from build123d import *

# Parameters (mm, degrees)
SKETCH_1_W          = 143
SKETCH_1_H          = 50
EXTRUDE_1_DEPTH     = 2
FILLET_1_R          = 3
CUT_EXTRUDE_1_DEPTH = 10
SKETCH_7_R          = 1.5
CUT_EXTRUDE_2_DEPTH = 10


with BuildPart() as part:
    # 草图1 → 凸台-拉伸1 (new body)
    with BuildSketch(Plane.XY):
        Rectangle(SKETCH_1_W, SKETCH_1_H)
    extrude(amount=EXTRUDE_1_DEPTH)

    # 圆角1
    fillet_1_edges = [part.edges().sort_by_distance(p)[0] for p in [
        (-71.5, 25, 1),
        (71.5, 25, 1),
        (71.5, -25, 1),
        (-71.5, -25, 1),
    ]]
    fillet(fillet_1_edges, radius=FILLET_1_R)

    # 草图2 → 切除-拉伸1 (cut)
    with BuildSketch(Plane.XY.offset(2)):
        with BuildLine():
            Line((5, 13), (5, -13))
            ThreePointArc((5, -13), (0, -18), (-5, -13))
            Line((-5, -13), (-5, 13))
            ThreePointArc((-5, 13), (0, 18), (5, 13))
        make_face()
        with BuildLine():
            Line((23, 13), (23, -13))
            ThreePointArc((23, -13), (18, -18), (13, -13))
            Line((13, -13), (13, 13))
            ThreePointArc((13, 13), (18, 18), (23, 13))
        make_face()
        with BuildLine():
            Line((41, 13), (41, -13))
            ThreePointArc((41, -13), (36, -18), (31, -13))
            Line((31, -13), (31, 13))
            ThreePointArc((31, 13), (36, 18), (41, 13))
        make_face()
        with BuildLine():
            Line((59, 13), (59, -13))
            ThreePointArc((59, -13), (54, -18), (49, -13))
            Line((49, -13), (49, 13))
            ThreePointArc((49, 13), (54, 18), (59, 13))
        make_face()
        with BuildLine():
            Line((-59, 13), (-59, -13))
            ThreePointArc((-59, -13), (-54, -18), (-49, -13))
            Line((-49, -13), (-49, 13))
            ThreePointArc((-49, 13), (-54, 18), (-59, 13))
        make_face()
        with BuildLine():
            Line((-41, 13), (-41, -13))
            ThreePointArc((-41, -13), (-36, -18), (-31, -13))
            Line((-31, -13), (-31, 13))
            ThreePointArc((-31, 13), (-36, 18), (-41, 13))
        make_face()
        with BuildLine():
            Line((-23, 13), (-23, -13))
            ThreePointArc((-23, -13), (-18, -18), (-13, -13))
            Line((-13, -13), (-13, 13))
            ThreePointArc((-13, 13), (-18, 18), (-23, 13))
        make_face()
    extrude(amount=-CUT_EXTRUDE_1_DEPTH, mode=Mode.SUBTRACT)

    # 草图7 → 切除-拉伸2 (cut)
    with BuildSketch(Plane(origin=(0, 0, 0), x_dir=(-1, 0, 0), z_dir=(0, 0, -1))):
        with Locations((-68.5, -3)):
            Circle(SKETCH_7_R)
        with Locations((-68.5, 17)):
            Circle(SKETCH_7_R)
    cut_extrude_2 = extrude(amount=-CUT_EXTRUDE_2_DEPTH, mode=Mode.SUBTRACT)

    # 镜向2: 切除-拉伸2 across plane
    add(cut_extrude_2.mirror(Plane.ZY), mode=Mode.SUBTRACT)


solid = part.part
Verification items for the finished model (mm, model axes). A direction names the side the tool comes from. Round coordinates to 2 decimals unless told otherwise and drop trailing zeros. Loops run counter-clockwise (first coordinate to the right, second up) from the corner with the lowest first, then second, coordinate; pieces in that order, holes last. Notation, with made-up numbers: (37, -7.75) - (65, -7.75) arc R13 ccw to (65, 1.25) - close; hole circle Ø4 at (13, 86.5). An arc over 180 degrees is marked (long way). Use a Markdown table: item, result. Add a question column.
1. Access from +Z, -Z, +X, -X, +Y, -Y to the whole of each face (thin tool, end or side, straight path). Record for faces 1 (the face through (-1, 23, 0)), 2 (the face through (36, 18, 1)).
2. Section check D-D, the plane x = 35. Record the boundary of the cut face in (y, z), plus the area to 3 significant figures.
3. Thickness scan on probe 1 along Y at (x, z) = (68.5, 1.2); probe 2 along Y at (x, z) = (36.5, 1.6); probe 3 along Y at (x, z) = (32, 1.5). Record the ranges inside material, lowest first. Write a range as [from, to].
4. Section check B-B, the plane z = 1.3. Give the number of separate pieces and of enclosed holes in the cut face, plus the area to 3 significant figures.
5. Release check for a two-part mould opening along Y. For faces 3 (the face through (70.6, -24.14, 1.01)), 4 (the face through (70.64, 24.1, 1.01)), 5 (the face through (54, 18, 1)) record: released by +Y, released by -Y, zero draft, split by the parting line, or undercut.
6. Section check A-A, the plane x = -18. Record the boundary of the cut face in (y, z).
Checks:
| question | item | result |
|---|---|---|
| 1 | face 1 | -Z, +X, -X, +Y, -Y |
| 1 | face 2 | +Z, -Z |
| 2 | outline | (-25, 0) - (-17.9, 0) - (-17.9, 2) - (-25, 2) - close; (17.9, 0) - (25, 0) - (25, 2) - (17.9, 2) - close |
| 2 | area | 28.4 mm^2 |
| 3 | probe 1 | y = [-25, -4.5], [-1.5, 15.5], [18.5, 25] |
| 3 | probe 2 | y = [-25, -17.97], [17.97, 25] |
| 3 | probe 3 | y = [-25, -16], [16, 25] |
| 4 | separate pieces | 1 |
| 4 | enclosed holes | 11 |
| 4 | area | 4,740 mm^2 |
| 5 | face 3 | released by -Y |
| 5 | face 4 | released by +Y |
| 5 | face 5 | undercut |
| 6 | outline | (-25, 0) - (-18, 0) - (-18, 2) - (-25, 2) - close; (18, 0) - (25, 0) - (25, 2) - (18, 2) - close |
